Part model, mm, in its own coordinate system. A direction names the side the tool comes from. Round coordinates to 2 decimals unless told otherwise and drop trailing zeros. Loops run counter-clockwise (first coordinate to the right, second up) from the corner with the lowest first, then second, coordinate; pieces in that order, holes last. Notation, with made-up numbers: M -26,24.25 L -14,24.25 A22 cw -14,52.25 Z; hole C 26.5,-23.5 d1. An arc over 180 degrees is marked long. Put each result on its own line as item: value. Start each with the question number.
1) Slice it at D-D on z = 7.5. Give the cut face in (x, y), then the cut area to 3 significant figures.
2) Drop flat-ended pins along their axis: pin 1 Ø1.5 at (y, z) = (48, 14) entering from +X; pin 2 Ø0.9 at (y, z) = (48, -2) entering from -X; pin 3 Ø1.5 at (y, z) = (48, 7) entering from -X. Give the stop position or say it passes through.
3) Which spindle directions (+Z, -Z, +X, -X, +Y, -Y) get a long thin tool onto all of the face, cutting with end or side? Do faces 4 (the flat face through (-35.335, 48, 10)), 5 (the flat face through (-25, 48, -3)), 6 (the flat face through (-17, 48, 0)), 7 (the flat face through (-14.335, 48, 34)). Say none if no direction does.
4) Probe line 1 along X through (y, z) = (49, 26); line 2 along Z through (x, y) = (-24.75, 49.05); line 3 along Z through (x, y) = (-19.25, 46.55). List the from-to ranges inside material, lowest first.
5) Slice it at C-C on z = 21.5. Give the cut face in (x, y), then the cut area to 3 significant figures.
6) Pull direction Z, two halves, no side cores. Call faces 1 (the cylindrical face through (-34.13, 47.74, 38.86)), 2 (the flat face through (-35.335, 48, 34)), 3 (the cylindrical face through (-33.826, 47.697, 26.396)): +Z half, -Z half, draft (parallel to the pull), parting line (faces both ways), or undercut.
7) Slice it at B-B on z = 26. Give the cut face in (x, y).
8) Slice it at A-A on y = 48.2. Give the cut face in (x, z), then the cut area to 3 significant figures.
```python
from build123d import *

# Parameters (mm, degrees)
CROQUIS1_W              = 11
CROQUIS1_H              = 3
SALIENTE_EXTRUIR1_DEPTH = 3
CROQUIS2_W              = 21
CROQUIS2_H              = 3
SALIENTE_EXTRUIR2_DEPTH = 40
CROQUIS3_R              = 9
CORTAR_EXTRUIR1_DEPTH   = 10
CROQUIS4_R              = 12
CROQUIS4_R_2            = 9
SALIENTE_EXTRUIR3_DEPTH = 3
REDONDEO1_R             = 4


with BuildPart() as part:
    # Croquis1 → Saliente-Extruir1 (new body)
    with BuildSketch(Plane.XY):
        with Locations((-24.835128068, 47.717862768)):
            Rectangle(CROQUIS1_W, CROQUIS1_H)
    extrude(amount=-SALIENTE_EXTRUIR1_DEPTH)

    # Croquis2 → Saliente-Extruir2 (add)
    with BuildSketch(Plane.XY):
        with Locations((-24.835128068, 47.717862768)):
            Rectangle(CROQUIS2_W, CROQUIS2_H)
    extrude(amount=SALIENTE_EXTRUIR2_DEPTH)

    # Croquis3 → Cortar-Extruir1 (cut)
    with BuildSketch(Plane.XZ.offset(-46.217862768)):
        with Locations((-24.835128068, 26)):
            Circle(CROQUIS3_R)
    extrude(amount=-CORTAR_EXTRUIR1_DEPTH, mode=Mode.SUBTRACT)

    # Croquis4 → Saliente-Extruir3 (add)
    with BuildSketch(Plane(origin=(0, 46.217862768, 0), x_dir=(-1, 0, 0), z_dir=(0, -1, 0))):
        with Locations((24.835128068, -26)):
            Circle(CROQUIS4_R)
        with Locations((24.835128068, -26)):
            Circle(CROQUIS4_R_2, mode=Mode.SUBTRACT)
    extrude(amount=-SALIENTE_EXTRUIR3_DEPTH)

    # Redondeo1
    redondeo1_edges = [part.edges().sort_by_distance(p)[0] for p in [
        (-35.335128068, 47.717862768, 40),
        (-14.335128068, 47.717862768, 40),
    ]]
    fillet(redondeo1_edges, radius=REDONDEO1_R)


solid = part.part
```
Recorded:
1. outline: M -35.34,46.22 L -14.34,46.22 L -14.34,49.22 L -35.34,49.22 Z
1. area: 63.0 mm2
2. pin 1: stops at x = -14.34
2. pin 2: stops at x = -30.34
2. pin 3: stops at x = -35.34
3. face 4: -Z, -X, +Y, -Y
3. face 5: -Z, +X, -X, +Y, -Y
3. face 6: -Z, +X, +Y, -Y
3. face 7: +Z, +X, +Y, -Y
4. line 1: x = -36.84 to -33.84, -15.84 to -12.84
4. line 2: z = -3 to 17, 35 to 40
4. line 3: z = 0 to 18.94, 33.06 to 40
5. outline: M -35.96,46.22 L -32.63,46.22 L -32.63,49.22 L -35.96,49.22 Z; M -17.04,46.22 L -13.71,46.22 L -13.71,49.22 L -17.04,49.22 Z
5. area: 20.0 mm2
6. face 1: +Z half
6. face 2: draft
6. face 3: undercut
7. outline: M -36.84,46.22 L -33.84,46.22 L -33.84,49.22 L -36.84,49.22 Z; M -15.84,46.22 L -12.84,46.22 L -12.84,49.22 L -15.84,49.22 Z
8. outline: M -35.34,0 L -30.34,0 L -30.34,-3 L -19.34,-3 L -19.34,0 L -14.34,0 L -14.34,20.19 A12 ccw -14.34,31.81 L -14.34,36 A4 ccw -18.34,40 L -31.34,40 A4 ccw -35.34,36 L -35.34,31.81 A12 ccw -35.34,20.19 Z; hole C -24.84,26 d18
8. area: 635 mm2
